Geometry: final body of the model. Coordinates: model frame, mm. Give positions to 0.01 mm unless a question says otherwise; leave off trailing zeros. Loops run counter-clockwise (first coordinate to the right, second up) from the corner with the lowest first, then second, coordinate; pieces in that order, holes last. Notation, with made-up numbers: (59, 11) - (100, 11) arc R25 cw to (100, 26) - close; hole circle Ø4 at (-2, 79.5). An arc over 180 degrees is marked (long way). Answer in a Markdown table with one row per item.
Autodesk Inventor part; units mm, degrees
ref_plane "YZ Plane" through (0, 0, 0) normal (1, 0, 0) x (0, 1, 0)
ref_plane "XZ Plane" through (0, 0, 0) normal (0, 1, 0) x (-1, 0, 0)
ref_plane "XY Plane" through (0, 0, 0) normal (0, 0, 1) x (1, 0, 0)
sketch "Sketch1" plane through (0, 0, 0) normal (0, 1, 0) x (-1, 0, 0)
  line L0 (-12.5, 5) -> (12.5, 5)
  line L1 (12.5, 5) -> (12.5, -5)
  line L2 (12.5, -5) -> (-12.5, -5)
  line L3 (-12.5, -5) -> (-12.5, 5)
  circle A0 centre (10.5, 3) radius 1
  circle A1 centre (10.5, -3) radius 1
  circle A2 centre (-10.5, 3) radius 1
  circle A3 centre (-10.5, -3) radius 1
  point P0 (0, 0)
  point P1 (0, 0)
  dimension "d0" = 25
  dimension "d1" = 10
  dimension "d3" = 2
  dimension "d4" = 2
  dimension "d5" = 2
  dimension "d6" = 2
  dimension "d7" = 2
  dimension "d8" = 2
  dimension "d9" = 2
  dimension "d10" = 2
  dimension "d13" = 2
  dimension "d14" = 2
  dimension "d15" = 2
  dimension "d16" = 2
  dimension "d17" = 6
  dimension "d18" = 21
extrude "Extrusion1" add sketch "Sketch1" along normal mid plane 2
properties part number "Plat"
Q1. First-contact query: pin 1 (3 mm diameter, centred on x = -10.5, z = -3, fed in from +Y); pin 2 (1.2 mm diameter, centred on x = -10.5, z = 3, fed in from +Y). Flat tips, straight axial feed; report the tip coordinate or a pass-through.
Check values:
| item | result |
|---|---|
| pin 1 | y = 1 |
| pin 2 | through |
Q2. Cut plane B-B (x = -10.5). Output: boundary loops of the cut face in (y, z).
Check values:
| item | result |
|---|---|
| outline | (-1, -5) - (1, -5) - (1, -4) - (-1, -4) - close; (-1, -2) - (1, -2) - (1, 2) - (-1, 2) - close; (-1, 4) - (1, 4) - (1, 5) - (-1, 5) - close |
Q3. Cut plane C-C (y = 0.45). Output: boundary loops of the cut face in (x, z).
Check values:
| item | result |
|---|---|
| outline | (-12.5, -5) - (12.5, -5) - (12.5, 5) - (-12.5, 5) - close; hole circle Ø2 at (-10.5, -3); hole circle Ø2 at (-10.5, 3); hole circle Ø2 at (10.5, -3); hole circle Ø2 at (10.5, 3) |
Q4. Material intervals for line 1 along Z through (x, y) = (10.5, -0.55); line 2 along X through (y, z) = (0.4, 2.75); line 3 along X through (y, z) = (0.15, -2.5), sorted ascending.
Check values:
| item | result |
|---|---|
| line 1 | -5 to -4, -2 to 2, 4 to 5 |
| line 2 | -12.5 to -11.47, -9.53 to 9.53, 11.47 to 12.5 |
| line 3 | -12.5 to -11.37, -9.63 to 9.63, 11.37 to 12.5 |
Q5. Draft query along Z for faces 1 (the flat face through (-12.5, 0, 0)), 2 (the cylindrical face through (11.3, 0, 3.6)), 3 (the flat face through (0, 0, -5)), 4 (the cylindrical face through (-9.7, 0, 3.6)). Return one class per face: pulls with the +Z half, pulls with the -Z half, needs draft (parallel to the pull), parting line crosses it, or undercut.
Check values:
| item | result |
|---|---|
| face 1 | needs draft |
| face 2 | undercut |
| face 3 | pulls with the -Z half |
| face 4 | undercut |
Q6. Cut plane A-A (z = -3). Output: boundary loops of the cut face in (x, y).
Check values:
| item | result |
|---|---|
| outline | (-12.5, -1) - (-11.5, -1) - (-11.5, 1) - (-12.5, 1) - close; (-9.5, -1) - (9.5, -1) - (9.5, 1) - (-9.5, 1) - close; (11.5, -1) - (12.5, -1) - (12.5, 1) - (11.5, 1) - close |
